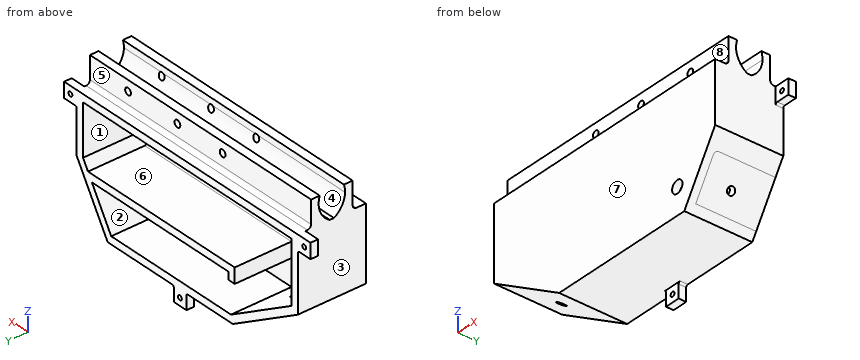
```python
from build123d import *

# Parameters (mm, degrees)
SKETCH1_W            = 350
SKETCH1_H            = 160
SKETCH1_W_2          = 330
SKETCH1_H_2          = 140
BOSS_EXTRUDE1_DEPTH  = 80
SKETCH2_W            = 350
SKETCH2_H            = 160
BOSS_EXTRUDE2_DEPTH  = 10
SKETCH3_W            = 240
SKETCH3_H            = 10
BOSS_EXTRUDE3_DEPTH  = 80
SKETCH4_R            = 8.25
CUT_EXTRUDE1_DEPTH   = 10
SKETCH5_W            = 10
SKETCH5_H            = 80
BOSS_EXTRUDE4_DEPTH  = 10
SKETCH6_W            = 35
SKETCH6_H            = 55
BOSS_EXTRUDE5_DEPTH  = 350
CUT_EXTRUDE2_DEPTH   = 377.994694923
SKETCH8_R            = 4.55
CUT_EXTRUDE3_DEPTH   = 222.599300704
SKETCH9_W            = 20
SKETCH9_H            = 20
SKETCH9_R            = 3.05
BOSS_EXTRUDE7_DEPTH  = 10
FILLET1_R            = 5
CUT_EXTRUDE5_DEPTH   = 244.618554386
SKETCH13_W           = 120.654432285
SKETCH13_H           = 90
BOSS_EXTRUDE8_DEPTH  = 10
CUT_EXTRUDE8_DEPTH   = 244.618554386
SKETCH15_W           = 93.792566681
SKETCH15_H           = 90
BOSS_EXTRUDE9_DEPTH  = 10
SKETCH16_W           = 20
SKETCH16_H           = 20
SKETCH16_R           = 3.05
BOSS_EXTRUDE10_DEPTH = 10
SKETCH17_R           = 5
CUT_EXTRUDE9_DEPTH   = 10
SKETCH18_R           = 6
CUT_EXTRUDE10_DEPTH  = 10
FILLET2_R            = 2.5


with BuildPart() as part:
    # Sketch1 → Boss-Extrude1 (new body)
    with BuildSketch(Plane(origin=(0, 0, 0), x_dir=(1, 0, 0), z_dir=(0, 1, 0))):
        Rectangle(SKETCH1_W, SKETCH1_H)
        Rectangle(SKETCH1_W_2, SKETCH1_H_2, mode=Mode.SUBTRACT)
    extrude(amount=BOSS_EXTRUDE1_DEPTH)

    # Sketch2 → Boss-Extrude2 (add)
    with BuildSketch(Plane.XZ):
        Rectangle(SKETCH2_W, SKETCH2_H)
    extrude(amount=BOSS_EXTRUDE2_DEPTH)

    # Sketch3 → Boss-Extrude3 (add)
    with BuildSketch(Plane(origin=(0, 0, 0), x_dir=(1, 0, 0), z_dir=(0, 1, 0))):
        with Locations((45, 15)):
            Rectangle(SKETCH3_W, SKETCH3_H)
    extrude(amount=BOSS_EXTRUDE3_DEPTH)

    # Sketch4 → Cut-Extrude1 (cut)
    with BuildSketch(Plane.XZ.offset(10)):
        with Locations(Location((115, -45, 0), (0, 0, 270))):
            Circle(SKETCH4_R)
    extrude(amount=-CUT_EXTRUDE1_DEPTH, mode=Mode.SUBTRACT)

    # Sketch5 → Boss-Extrude4 (add)
    with BuildSketch(Plane(origin=(0, 0, -20), x_dir=(-1, 0, 0), z_dir=(0, 0, -1))):
        with Locations((70, 40)):
            Rectangle(SKETCH5_W, SKETCH5_H)
    extrude(amount=BOSS_EXTRUDE4_DEPTH)

    # Sketch6 → Boss-Extrude5 (add)
    with BuildSketch(Plane.ZY.offset(175)):
        with Locations((97.5, 35)):
            Rectangle(SKETCH6_W, SKETCH6_H)
    extrude(amount=-BOSS_EXTRUDE5_DEPTH)

    # Sketch7 → Cut-Extrude2 (cut, through all)
    with BuildSketch(Plane.ZY.offset(175)):
        with BuildLine():
            Line((80, 32.25), (80, 37.75))
            ThreePointArc((80, 37.75), (90.572772871, 48.370529591), (104.96357244, 52.551924426))
            add(Edge.make_bspline(
                [(105.036319557, 17.552000028), (130.036265556, 17.603962255), (129.999891997, 35.103924454), (129.963518438, 52.603886653), (104.96357244, 52.551924426)],
                knots=[1.570796327, 1.570796327, 1.570796327, 3.141592654, 3.141592654, 4.71238898, 4.71238898, 4.71238898], degree=2, weights=[1, 0.707106781, 1, 0.707106781, 1]))
            ThreePointArc((105.036319557, 17.552000028), (90.621814813, 21.670798719), (80, 32.25))
        make_face()
    extrude(amount=-CUT_EXTRUDE2_DEPTH, mode=Mode.SUBTRACT)

    # Sketch8 → Cut-Extrude3 (cut, through all)
    with BuildSketch(Plane(origin=(0, 62.5, 0), x_dir=(1, 0, 0), z_dir=(0, 1, 0))):
        with Locations(Location((-35, -101, 0), (0, 0, 242.51146341))):
            Circle(SKETCH8_R)
        with Locations(Location((36.6, -101, 0), (0, 0, 242.51146341))):
            Circle(SKETCH8_R)
        with Locations(Location((114.7, -101, 0), (0, 0, 242.51146341))):
            Circle(SKETCH8_R)
    extrude(amount=-CUT_EXTRUDE3_DEPTH, mode=Mode.SUBTRACT)

    # Sketch9 → Boss-Extrude7 (add)
    # profile 1 of 2: a face of its own
    with BuildSketch(Plane(origin=(0, 80, 0), x_dir=(1, 0, 0), z_dir=(0, 1, 0))):
        with Locations((185, -70)):
            Rectangle(SKETCH9_W, SKETCH9_H)
        with Locations(Location((185, -70, 0), (0, 0, 270))):
            Circle(SKETCH9_R, mode=Mode.SUBTRACT)
    # profile 2 of 2: a face of its own
    with BuildSketch(Plane(origin=(0, 80, 0), x_dir=(1, 0, 0), z_dir=(0, 1, 0))):
        with Locations((-185, -70)):
            Rectangle(SKETCH9_W, SKETCH9_H)
        with Locations(Location((-185, -70, 0), (0, 0, 90))):
            Circle(SKETCH9_R, mode=Mode.SUBTRACT)
    extrude(amount=-BOSS_EXTRUDE7_DEPTH)

    # Fillet1
    fillet1_edges = [part.edges().sort_by_distance(p)[0] for p in [
        (45, 0, -10),
        (50, 0, -20),
        (0, 7.5, 80),
        (0, 62.5, 80),
    ]]
    fillet(fillet1_edges, radius=FILLET1_R)

    # Sketch12 → Cut-Extrude5 (cut, through all)
    with BuildSketch(Plane(origin=(0, 80, 0), x_dir=(1, 0, 0), z_dir=(0, 1, 0))):
        Polygon((-72.01506271, 80), (-175, 17.138288908), (-175, 80), align=None)
    extrude(amount=-CUT_EXTRUDE5_DEPTH, mode=Mode.SUBTRACT)

    # Sketch13 → Boss-Extrude8 (add)
    with BuildSketch(Plane(origin=(-55.124817516, 0, -90.309757345), x_dir=(-0.8535528727753664, 0, 0.5210062316104475), z_dir=(-0.5210062316104475, 0, -0.8535528727753664))):
        with Locations((80.115381273, 35)):
            Rectangle(SKETCH13_W, SKETCH13_H)
    extrude(amount=-BOSS_EXTRUDE8_DEPTH)

    # Sketch14 → Cut-Extrude8 (cut, through all)
    with BuildSketch(Plane(origin=(0, 80, 0), x_dir=(1, 0, 0), z_dir=(0, 1, 0))):
        Polygon((126.04036801, 80), (175, 0), (175, 80), align=None)
    extrude(amount=-CUT_EXTRUDE8_DEPTH, mode=Mode.SUBTRACT)

    # Sketch15 → Boss-Extrude9 (add)
    with BuildSketch(Plane(origin=(127.315471061, 0, -77.916482622), x_dir=(-0.5219990637024984, 0, -0.8529460577866077), z_dir=(0.8529460577866077, 0, -0.5219990637024984))):
        with Locations((-44.453552808, 35)):
            Rectangle(SKETCH15_W, SKETCH15_H)
    extrude(amount=-BOSS_EXTRUDE9_DEPTH)

    # Sketch16 → Boss-Extrude10 (add)
    with BuildSketch(Plane(origin=(0, 80, 0), x_dir=(1, 0, 0), z_dir=(0, 1, 0))):
        with Locations((11.381009241, 90)):
            Rectangle(SKETCH16_W, SKETCH16_H)
        with Locations(Location((11.718047049, 90, 0), (0, 0, 270))):
            Circle(SKETCH16_R, mode=Mode.SUBTRACT)
    extrude(amount=-BOSS_EXTRUDE10_DEPTH)

    # Sketch17 → Cut-Extrude9 (cut)
    with BuildSketch(Plane(origin=(127.315471061, 0, -77.916482622), x_dir=(-0.5219990637024984, 0, -0.8529460577866076), z_dir=(0.8529460577866077, 0, -0.5219990637024985))):
        with Locations((-36.349836148, 35)):
            Circle(SKETCH17_R)
    extrude(amount=-CUT_EXTRUDE9_DEPTH, mode=Mode.SUBTRACT)

    # Sketch18 → Cut-Extrude10 (cut)
    with BuildSketch(Plane(origin=(-55.124817516, 0, -90.309757345), x_dir=(-0.8535528727753664, 0, 0.5210062316104476), z_dir=(-0.5210062316104476, 0, -0.8535528727753664))):
        with Locations((79.494288209, 35.423286216)):
            Circle(SKETCH18_R)
    extrude(amount=-CUT_EXTRUDE10_DEPTH, mode=Mode.SUBTRACT)

    # Fillet2
    fillet2_edges = [part.edges().sort_by_distance(p)[0] for p in [
        (175, 75, 60),
        (-175, 75, 60),
        (1.381009241, 75, -80),
        (21.381009241, 75, -80),
    ]]
    fillet(fillet2_edges, radius=FILLET2_R)


solid = part.part
```
CAD build for the part. Positions are in the model's coordinates, mm. Face numbers are marked on the shaded views. A direction names the side the tool comes from. Round coordinates to 2 decimals unless told otherwise and drop trailing zeros. Loops run counter-clockwise (first coordinate to the right, second up) from the corner with the lowest first, then second, coordinate; pieces in that order, holes last. Notation, with made-up numbers: M -9.75,74.5 L 48.25,74.5 A10 ccw 48.25,85.5 Z; hole C -39.75,78 d1. An arc over 180 degrees is marked long. Return JSON: item names as keys, results as strings. Group by question number.
(1) Saw through at A-A, the plane z = 14.5. List the corners of the cut face in (x, y).
(2) Mould opens along X. For the marked faces 1, 2, 3 and 4 say: +X half, -X half, draft (parallel to the pull), parting line (faces both ways), or undercut.
(3) Wall check: probe 1 along Z at (x, y) = (-35, 13); probe 2 along X at (y, z) = (47.5, 45.5); probe 3 along X at (y, z) = (77.5, -90). Give the ranges that are in metal, low to high. Write a range as [from, to].
(4) Drop flat-ended pins along their axis: P1, Ø10, axis at y = 32, z = 30, coming from the -X side; P2, Ø9, axis at x = 60, z = 107, coming from the +Y side; P3, Ø3, axis at x = 22.5, z = -64, coming from the +Y side. Give the stop position or say it passes through.
(5) Tool access for the marked faces 5, 6, 7 and 8: list every direction of +Z, -Z, +X, -X, +Y, -Y with a clear straight run to the whole face (end or side of a thin tool).
(6) Saw through at B-B, the plane z = 101. Give the number of separate pieces and of enclosed holes in the cut face, and give its area (3 significant figures).
Answer list:
{
 "1": {"outline": "M -175,-10 L 175,-10 L 175,80 L 165,80 L 165,0 L -165,0 L -165,80 L -175,80 Z"},
 "2": {"face 1": "undercut", "face 2": "undercut", "face 3": "-X half", "face 4": "draft"},
 "3": {"probe 1": "[-80, -70], [-20, -10], [70, 96.45], [105.55, 115]", "probe 2": "[-175, -165], [165, 175]", "probe 3": "[1.38, 8.67], [14.77, 21.38]"},
 "4": {"P1": "x = -175", "P2": "y = 62.5", "P3": "y = 0"},
 "5": {"face 5": "+Z, +X, -X, +Y", "face 6": "+Y", "face 7": "+Z, -Z, +X, -X, -Y", "face 8": "+Z, +X, -X, -Y"},
 "6": {"separate pieces": "8", "enclosed holes": "0", "area": "6,700 mm2"}
}
